Verification items for the finished model (mm, model axes). Face numbers are marked on the shaded views. A direction names the side the tool comes from. Round coordinates to 2 decimals unless told otherwise and drop trailing zeros. Write each loop counter-clockwise with the first axis right and the second up, starting at its lowest first coordinate (ties: lowest second). Pieces come first, ordered by that corner, then holes. Notation, with made-up numbers: (45, 16.25) -> (83, 16.25) arc R27 ccw to (83, 38.25) -> close; hole circle Ø2 at (62.25, 35.5). An arc over 180 degrees is marked (long way). Answer as a JSON object with one key per item and string values. Group by question number.
(1) Draft check along X on the marked faces 4 and 5. Enter one of: released by +X, released by -X, zero draft, split by the parting line, or undercut.
(2) Scan lines: L1, parallel to Z at x = 0, y = 5.1; L2, parallel to X at y = 0.55, z = 0; L3, parallel to Z at x = 18, y = 1.25. Record each from-to range of solid material in increasing order. Write a range as from..to.
(3) Sectioned sample at C-C on y = 3. Record the cut outline in (x, z).
(4) Set-up check for the marked faces 1, 2 and 3: record each of +Z, -Z, +X, -X, +Y, -Y from which the full face is reachable in a straight line by a thin tool's end or side.
(5) Sectioned sample at A-A on x = -18. Record the cut outline in (y, z), and give its area (3 significant figures).
(6) Sectioned sample at D-D on x = -4.5. Record the cut outline in (y, z), and give its area (3 significant figures).
(7) Gauge pin test, flat ends, axial feed: pin 1 Ø2.5 at (x, z) = (-17.5, -2) entering from +Y; pin 2 Ø7.5 at (x, z) = (0, -22) entering from +Y; pin 3 Ø1.6 at (x, y) = (13.5, 0.5) entering from -Z. Record the tip position at first contact, or that the pin passes through.
(8) Sectioned sample at B-B on z = 0. Record the cut outline in (x, y).
```python
from build123d import *

# Parameters (mm, degrees)
SKETCH1_W           = 17
SKETCH1_H           = 55
SKETCH1_R           = 7.55
SKETCH1_W_2         = 14
SKETCH1_H_2         = 9
SKETCH1_R_2         = 1.5
BOSS_EXTRUDE1_DEPTH = 2
BOSS_EXTRUDE2_START = 2
SKETCH1_4_W         = 17
SKETCH1_4_H         = 55
SKETCH1_4_R         = 7.55
BOSS_EXTRUDE2_DEPTH = 1.838
BOSS_EXTRUDE3_START = 3.838
SKETCH1_5_W         = 17
SKETCH1_5_H         = 55
SKETCH1_5_R         = 7.55
BOSS_EXTRUDE3_DEPTH = 2.25
SKETCH3_R           = 3
CUT_EXTRUDE1_DEPTH  = 7.088


with BuildPart() as part:
    # Sketch1 → Boss-Extrude1 (new body)
    with BuildSketch(Plane(origin=(0, 0, 0), x_dir=(1, 0, 0), z_dir=(0, 1, 0))):
        Rectangle(SKETCH1_W, SKETCH1_H)
        with Locations((0, -18.8625)):
            Circle(SKETCH1_R, mode=Mode.SUBTRACT)
        with Locations((0, 18.8625)):
            Circle(SKETCH1_R, mode=Mode.SUBTRACT)
        with Locations((15.5, 0)):
            Rectangle(SKETCH1_W_2, SKETCH1_H_2)
        with Locations((18, 0)):
            Circle(SKETCH1_R_2, mode=Mode.SUBTRACT)
        with Locations((-15.5, 0)):
            Rectangle(SKETCH1_W_2, SKETCH1_H_2)
        with Locations((-18, 0)):
            Circle(SKETCH1_R_2, mode=Mode.SUBTRACT)
        with Locations((0, -18.8625)):
            Circle(SKETCH1_R)
        with Locations((0, 18.8625)):
            Circle(SKETCH1_R)
    extrude(amount=BOSS_EXTRUDE1_DEPTH)

    # Sketch1<4> → Boss-Extrude2 (add)
    with BuildSketch(Plane(origin=(0, 0, 0), x_dir=(1, 0, 0), z_dir=(0, 1, 0)).offset(BOSS_EXTRUDE2_START)):
        Rectangle(SKETCH1_4_W, SKETCH1_4_H)
        with Locations((0, -18.8625)):
            Circle(SKETCH1_4_R, mode=Mode.SUBTRACT)
        with Locations((0, 18.8625)):
            Circle(SKETCH1_4_R, mode=Mode.SUBTRACT)
        with Locations((0, -18.8625)):
            Circle(SKETCH1_4_R)
        with Locations((0, 18.8625)):
            Circle(SKETCH1_4_R)
    extrude(amount=BOSS_EXTRUDE2_DEPTH)

    # Sketch1<5> → Boss-Extrude3 (add)
    with BuildSketch(Plane(origin=(0, 0, 0), x_dir=(1, 0, 0), z_dir=(0, 1, 0)).offset(BOSS_EXTRUDE3_START)):
        Rectangle(SKETCH1_5_W, SKETCH1_5_H)
        with Locations((0, -18.8625)):
            Circle(SKETCH1_5_R, mode=Mode.SUBTRACT)
        with Locations((0, 18.8625)):
            Circle(SKETCH1_5_R, mode=Mode.SUBTRACT)
    extrude(amount=BOSS_EXTRUDE3_DEPTH)

    # Sketch3 → Cut-Extrude1 (cut, through all)
    with BuildSketch(Plane.XZ):
        with Locations((0, -18.8625)):
            Circle(SKETCH3_R)
        with Locations((0, 18.8625)):
            Circle(SKETCH3_R)
    extrude(amount=-CUT_EXTRUDE1_DEPTH, mode=Mode.SUBTRACT)


solid = part.part
```
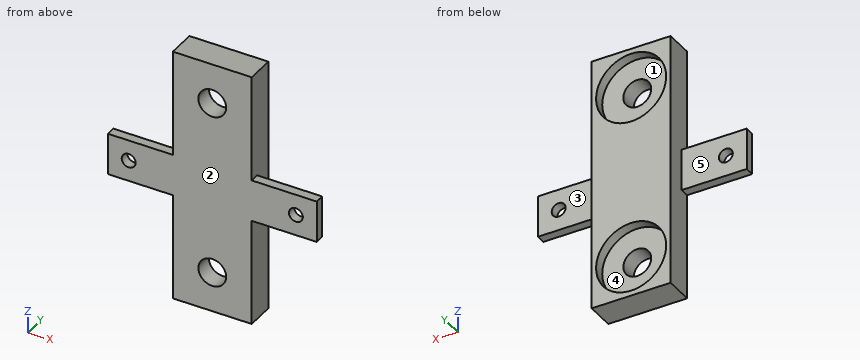
Computed values:
{
 "1": {"face 4": "undercut", "face 5": "zero draft"},
 "2": {"L1": "-27.5..-26.41, -11.31..11.31, 26.41..27.5", "L2": "-22.5..-19.5, -16.5..16.5, 19.5..22.5", "L3": "-4.5..-1.5, 1.5..4.5"},
 "3": {"outline": "(-8.5, -27.5) -> (8.5, -27.5) -> (8.5, 27.5) -> (-8.5, 27.5) -> close; hole circle Ø6 at (0, -18.86); hole circle Ø6 at (0, 18.86)"},
 "4": {"face 1": "+Y", "face 2": "+Z, -Z, +X, -X, -Y", "face 3": "+Z, -Z, +X, +Y"},
 "5": {"outline": "(0, -4.5) -> (2, -4.5) -> (2, -1.5) -> (0, -1.5) -> close; (0, 1.5) -> (2, 1.5) -> (2, 4.5) -> (0, 4.5) -> close", "area": "12.0 mm2"},
 "6": {"outline": "(0, -27.5) -> (6.09, -27.5) -> (6.09, -24.92) -> (3.84, -24.92) -> (3.84, -12.8) -> (6.09, -12.8) -> (6.09, 12.8) -> (3.84, 12.8) -> (3.84, 24.92) -> (6.09, 24.92) -> (6.09, 27.5) -> (0, 27.5) -> close", "area": "280 mm2"},
 "7": {"pin 1": "y = 2", "pin 2": "y = 3.84", "pin 3": "z = -4.5"},
 "8": {"outline": "(-22.5, 0) -> (-19.5, 0) -> (-19.5, 2) -> (-22.5, 2) -> close; (-16.5, 0) -> (16.5, 0) -> (16.5, 2) -> (8.5, 2) -> (8.5, 6.09) -> (-8.5, 6.09) -> (-8.5, 2) -> (-16.5, 2) -> close; (19.5, 0) -> (22.5, 0) -> (22.5, 2) -> (19.5, 2) -> close"}
}
